Autodesk Fusion 360 part; units mm, degrees
sketch "スケッチ1" plane through (0, 0, 0) normal (0, 0, 1) x (1, 0, 0)
  line L0 (-15.5, 115) -> (-74.5, 115)
  line L1 (-74.5, 115) -> (-74.5, -115)
  line L2 (-74.5, -115) -> (-15.5, -115)
  line L3 (74.5, -105) -> (74.5, 105)
  line L4 (68.0217, 105) -> (-74.5, -115) construction
  line L5 (-74.5, 115) -> (68.0217, -105) construction
  line L6 (-15.5, 115) -> (-15.5, 105)
  line L7 (-15.5, 105) -> (74.5, 105)
  line L8 (-15.5, -115) -> (-15.5, -105)
  line L9 (-15.5, -105) -> (74.5, -105)
  dimension "d2" = 230
extrude "押し出し1" add sketch "スケッチ1" along normal blind 6
chamfer "面取り1" distance 20 angle 45 2 edges at (-74.5, -115, 3) (-74.5, 115, 3)
sketch "スケッチ2" plane through (0, 0, 6) normal (0, 0, 1) x (-1, 0, 0)
  line L0 (54.5, -115) -> (74.5, -95)
  line L1 (74.5, -95) -> (74.5, 95)
  line L2 (74.5, 95) -> (54.5, 115)
  line L3 (54.5, 115) -> (15.5, 115)
  line L4 (15.5, 115) -> (15.5, 105)
  line L5 (15.5, 105) -> (-74.5, 105)
  line L6 (-74.5, 105) -> (-74.5, -105)
  line L7 (-74.5, -105) -> (15.5, -105)
  line L8 (15.5, -105) -> (15.5, -115)
  line L9 (15.5, -115) -> (54.5, -115)
  line L10 (-74.5, -105) -> (-34.5, -105)
  line L11 (-34.5, -105) -> (-34.5, -60)
  line L12 (-34.5, -60) -> (-74.5, -60)
  line L13 (-74.5, -60) -> (-74.5, -105)
  line L14 (-34.5, -60) -> (-34.5, 0)
  line L15 (-34.5, 0) -> (-34.5, 60)
  point P0 (-34.5, -60)
  point P1 (-34.5, 0)
  point P2 (-34.5, 60)
  dimension "d10" = 40
  dimension "d11" = 45
  dimension "d12" = 60
  dimension "d13" = 60
hole "穴1" at (34.5, 60, 6) at (34.5, 0, 6) at (34.5, -60, 6) direction (0, 0, -1) diameter 18 end through all
CAD build for the part. Positions are in the model's coordinates, mm. A direction names the side the tool comes from. Give positions to 0.01 mm unless a question says otherwise; leave off trailing zeros. Order: outer loops, then holes, each group sorted by start corner. A loop starts at its lowest first (then second) coordinate and runs counter-clockwise, first axis right, second up.
(1) Saw through at A-A, the plane x = 34.5. Give the cut face in (y, z).
(2) Saw through at C-C, the plane z = 1.9. Give the cut face in (x, y).
(3) Tool access for faces 1 (the flat face through (29, -105, 3)), 2 (the flat face through (29, 105, 3)), 3 (the flat face through (-1, 2, 6)): list every direction of +Z, -Z, +X, -X, +Y, -Y with a clear straight run to the whole face (end or side of a thin tool).
(4) Flat gauge pins, fed straight in: pin 1 (1.5 mm diameter, centred on x = 44, z = 2, fed in from +Y); pin 2 (1.8 mm diameter, centred on x = 20.5, z = 4.5, fed in from -Y); pin 3 (1.8 mm diameter, centred on y = 109, z = 4, fed in from +X); pin 4 (23.5 mm diameter, centred on x = 34.5, y = 0, fed in from +Z). Where does each tip first touch, or does it go through?
(5) Saw through at B-B, the plane y = 0. Give the cut face in (x, z), then the cut area to 3 significant figures.
(6) Saw through at D-D, the plane y = 66. Give the cut face in (x, z).
(7) Mould opens along Y. For faces 4 (the flat face through (74.5, -1, 3)), 5 (the cylindrical face through (26.91, 55.16, 2.96)), 6 (the flat face through (-64.4, 105.1, 3)), 7 (the flat face through (-35, -115, 3)) say: released by +Y, released by -Y, zero draft, split by the parting line, or undercut.
(8) Drill centre lines: L1, parallel to Y at x = 34.5, z = 2.85; L2, parallel to X at y = 0, z = 4.25; L3, parallel to Y at x = 36, z = 5.6. Where is each one in solid material? Low to high.
Results found:
1. outline: (-105, 0) - (-69, 0) - (-69, 6) - (-105, 6) - close; (-51, 0) - (-9, 0) - (-9, 6) - (-51, 6) - close; (9, 0) - (51, 0) - (51, 6) - (9, 6) - close; (69, 0) - (105, 0) - (105, 6) - (69, 6) - close
2. outline: (-74.5, -95) - (-54.5, -115) - (-15.5, -115) - (-15.5, -105) - (74.5, -105) - (74.5, 105) - (-15.5, 105) - (-15.5, 115) - (-54.5, 115) - (-74.5, 95) - close; hole circle Ø18 at (34.5, -60); hole circle Ø18 at (34.5, 0); hole circle Ø18 at (34.5, 60)
3. face 1: +Z, -Z, +X, -Y
3. face 2: +Z, -Z, +X, +Y
3. face 3: +Z, +X, -X, +Y, -Y
4. pin 1: stops at y = 105
4. pin 2: stops at y = -105
4. pin 3: stops at x = -15.5
4. pin 4: stops at z = 6
5. outline: (-74.5, 0) - (25.5, 0) - (25.5, 6) - (-74.5, 6) - close; (43.5, 0) - (74.5, 0) - (74.5, 6) - (43.5, 6) - close
5. area: 786 mm2
6. outline: (-74.5, 0) - (27.79, 0) - (27.79, 6) - (-74.5, 6) - close; (41.21, 0) - (74.5, 0) - (74.5, 6) - (41.21, 6) - close
7. face 4: zero draft
7. face 5: undercut
7. face 6: released by +Y
7. face 7: released by -Y
8. L1: y = -105 to -69, -51 to -9, 9 to 51, 69 to 105
8. L2: x = -74.5 to 25.5, 43.5 to 74.5
8. L3: y = -105 to -68.87, -51.13 to -8.87, 8.87 to 51.13, 68.87 to 105
